Part model, mm, in its own coordinate system. A direction names the side the tool comes from. Coordinates: 2 decimals unless noted, no trailing zeros. Loops run counter-clockwise (first coordinate to the right, second up) from the corner with the lowest first, then second, coordinate; pieces in that order, holes last. Notation, with made-up numbers: (43.25, 51.5) - (67.25, 51.5) arc R13 ccw to (67.25, 75.5) - close; hole circle Ø8 at (-12.5, 14). An arc over 180 degrees is marked (long way). Use a Markdown table: item, result. Add a question column.
1. Wall check: probe 1 along X at (y, z) = (7.75, -19); probe 2 along X at (y, z) = (1.75, -3). Give the ranges that are in metal, low to high. Write a range as [from, to].
2. Drop flat-ended pins along their axis: pin 1 (1 mm diameter, centred on y = 0.5, z = 6.5, fed in from -X); pin 2 (0.5 mm diameter, centred on x = -2.5, y = 8, fed in from +Z); pin 3 (1 mm diameter, centred on x = 7.5, y = 8.5, fed in from +Z). Give the stop position or say it passes through.
3. Band-saw the part on B-B, the plane y = 4. Give the cut face in (x, z).
4. Band-saw the part on C-C, the plane x = 11.5. Give the cut face in (y, z).
5. Band-saw the part on A-A, the plane z = -16. Give the cut face in (x, y), plus the area to 3 significant figures.
6. 3-axis set-ups, long thin cutter, end or side, ignore diameter. For faces 4 (the flat face through (48.64, 4.36, 48.07)), 5 (the flat face through (45.543, 0.896, 46.075)), 6 (the cylindrical face through (-48.38, 0.342, 47.819)), 7 (the flat face through (0, 4, -63.184)), 8 (the flat face through (-45.543, 7.904, 46.075)): which of +Z, -Z, +X, -X, +Y, -Y reach the whole face in a straight line?
7. Pull direction Z, two halves, no side cores. Call faces 1 (the flat face through (45.543, 7.904, -46.075)), 2 (the cylindrical face through (-47.819, 0.342, -48.38)), 3 (the flat face through (-48.07, 4.36, 48.64)): pulls with the +Z half, pulls with the -Z half, needs draft (parallel to the pull), parting line crosses it, or undercut.
Autodesk Inventor part; units mm, degrees
ref_plane "작업 평면3" through (0, 4.4, 0) normal (0, -1, 0) x (1, 0, 0)
ref_plane "YZ Plane" through (0, 0, 0) normal (1, 0, 0) x (0, 1, 0)
ref_plane "XZ Plane" through (0, 0, 0) normal (0, 1, 0) x (-1, 0, 0)
sketch "스케치1" plane through (0, 0, 0) normal (0, 1, 0) x (-1, 0, 0)
  line L0 (-65.1838, 27) -> (-27, 65.1838)
  line L1 (-27, 65.1838) -> (27, 65.1838)
  line L2 (27, 65.1838) -> (65.1838, 27)
  line L3 (65.1838, 27) -> (65.1838, -27)
  line L4 (65.1838, -27) -> (27, -65.1838)
  line L5 (27, -65.1838) -> (-27, -65.1838)
  line L6 (-27, -65.1838) -> (-65.1838, -27)
  line L7 (-65.1838, -27) -> (-65.1838, 27)
  line L8 (68.3838, 28.3255) -> (68.3838, -28.3255)
  line L9 (68.3838, -28.3255) -> (28.3255, -68.3838)
  line L10 (28.3255, -68.3838) -> (-28.3255, -68.3838)
  line L11 (-28.3255, -68.3838) -> (-68.3838, -28.3255)
  line L12 (-68.3838, -28.3255) -> (-68.3838, 28.3255)
  line L13 (-68.3838, 28.3255) -> (-28.3255, 68.3838)
  line L14 (-28.3255, 68.3838) -> (28.3255, 68.3838)
  line L15 (28.3255, 68.3838) -> (68.3838, 28.3255)
  point P0 (0, 0)
  point P1 (0, 0)
  point P2 (0, 0)
  dimension "d0" = 54
  dimension "d1" = 3.2
extrude "돌출1" add sketch "스케치1" along normal blind 8.8 contours L0 L1 L2 L3 L4 L5 L6 L7 | L8 L9 L10 L11 L12 L13 L14 L15
sketch "스케치3" plane through (0, 0, 0) normal (0, -1, 0) x (1, 0, 0)
  line L0 (-26.8343, 64.7838) -> (26.8343, 64.7838)
  line L1 (26.8343, 64.7838) -> (64.7838, 26.8343)
  line L2 (64.7838, 26.8343) -> (64.7838, -26.8343)
  line L3 (64.7838, -26.8343) -> (26.8343, -64.7838)
  line L4 (26.8343, -64.7838) -> (-26.8343, -64.7838)
  line L5 (-26.8343, -64.7838) -> (-64.7838, -26.8343)
  line L6 (-64.7838, -26.8343) -> (-64.7838, 26.8343)
  line L7 (-64.7838, 26.8343) -> (-26.8343, 64.7838)
  line L8 (-27.6627, 66.7838) -> (27.6627, 66.7838)
  line L9 (27.6627, 66.7838) -> (66.7838, 27.6627)
  line L10 (66.7838, 27.6627) -> (66.7838, -27.6627)
  line L11 (66.7838, -27.6627) -> (27.6627, -66.7838)
  line L12 (27.6627, -66.7838) -> (-27.6627, -66.7838)
  line L13 (-27.6627, -66.7838) -> (-66.7838, -27.6627)
  line L14 (-66.7838, -27.6627) -> (-66.7838, 27.6627)
  line L15 (-66.7838, 27.6627) -> (-27.6627, 66.7838)
  line L16 (-28.3255, 68.3838) -> (28.3255, 68.3838)
  point P0 (0, 0)
  point P1 (0, 0)
  point P2 (0, 0)
  point P3 (0, 0)
  dimension "d9" = 2
  dimension "d144" = 1.6
extrude "돌출3" cut sketch "스케치3" against normal blind 1.2
sketch "스케치14" plane through (0, 0, 0) normal (0, -1, 0) x (1, 0, 0)
  line L0 (64.7838, 26.8343) -> (26.8343, 64.7838)
  line L1 (26.8343, 64.7838) -> (-26.8343, 64.7838)
  line L2 (-26.8343, 64.7838) -> (-64.7838, 26.8343)
  line L3 (-64.7838, 26.8343) -> (-64.7838, -26.8343)
  line L4 (-64.7838, -26.8343) -> (-26.8343, -64.7838)
  line L5 (-26.8343, -64.7838) -> (26.8343, -64.7838)
  line L6 (26.8343, -64.7838) -> (64.7838, -26.8343)
  line L7 (64.7838, -26.8343) -> (64.7838, 26.8343)
  point P0 (0, 0)
extrude "돌출16" cut sketch "스케치14" against normal blind 0.6
sketch "스케치15" plane through (0, 0.6, 0) normal (0, -1, 0) x (1, 0, 0)
  line L0 (-26.1716, 63.1838) -> (26.1716, 63.1838)
  line L1 (26.1716, 63.1838) -> (63.1838, 26.1716)
  line L2 (63.1838, 26.1716) -> (63.1838, -26.1716)
  line L3 (63.1838, -26.1716) -> (26.1716, -63.1838)
  line L4 (26.1716, -63.1838) -> (-26.1716, -63.1838)
  line L5 (-26.1716, -63.1838) -> (-63.1838, -26.1716)
  line L6 (-63.1838, -26.1716) -> (-63.1838, 26.1716)
  line L7 (-63.1838, 26.1716) -> (-26.1716, 63.1838)
  line L8 (-26.8343, 64.7838) -> (26.8343, 64.7838)
  point P0 (0, 0)
  point P1 (0, 0)
  dimension "d140" = 1.6
extrude "돌출17" cut sketch "스케치15" against normal up to surface (8.2 mm away)
ref_plane "작업 평면3" through (0, 4.4, 0) normal (0, -1, 0) x (1, 0, 0)
mirror "미러6" about plane through (0, 4.4, 0) normal (0, -1, 0) of "돌출3", "돌출16"
fillet "모깎기2" radius 1.2 16 edges at (0, 0, 68.3838) (-48.3546, 0, 48.3546) (-68.3838, 0, 0) (-48.3546, 0, -48.3546) (0, 0, -68.3838) (48.3546, 0, -48.3546) (68.3838, 0, 0) (48.3546, 0, 48.3546) (-48.3546, 8.8, 48.3546) (-68.3838, 8.8, 0) (-48.3546, 8.8, -48.3546) (0, 8.8, -68.3838) (48.3546, 8.8, -48.3546) (68.3838, 8.8, 0) (48.3546, 8.8, 48.3546) (0, 8.8, 68.3838)
properties part number "OV-PAM_ring_2"
Geometry check:
| question | item | result |
|---|---|---|
| 1 | probe 1 | x = [-68.37, -66.78], [-64.78, -63.18], [63.18, 64.78], [66.78, 68.37] |
| 1 | probe 2 | x = [-68.38, -63.18], [63.18, 68.38] |
| 2 | pin 1 | stops at x = -68.37 |
| 2 | pin 2 | stops at z = 68.37 |
| 2 | pin 3 | stops at z = 68.32 |
| 3 | outline | (-68.38, -28.33) - (-28.33, -68.38) - (28.33, -68.38) - (68.38, -28.33) - (68.38, 28.33) - (28.33, 68.38) - (-28.33, 68.38) - (-68.38, 28.33) - close; hole (-63.18, -26.17) - (-26.17, -63.18) - (26.17, -63.18) - (63.18, -26.17) - (63.18, 26.17) - (26.17, 63.18) - (-26.17, 63.18) - (-63.18, 26.17) - close |
| 4 | outline | (0, -67.18) arc R1.2 ccw to (1.2, -68.38) - (7.6, -68.38) arc R1.2 ccw to (8.8, -67.18) - (8.8, -66.78) - (7.6, -66.78) - (7.6, -64.78) - (8.2, -64.78) - (8.2, -63.18) - (0.6, -63.18) - (0.6, -64.78) - (1.2, -64.78) - (1.2, -66.78) - (0, -66.78) - close; (0, 66.78) - (1.2, 66.78) - (1.2, 64.78) - (0.6, 64.78) - (0.6, 63.18) - (8.2, 63.18) - (8.2, 64.78) - (7.6, 64.78) - (7.6, 66.78) - (8.8, 66.78) - (8.8, 67.18) arc R1.2 ccw to (7.6, 68.38) - (1.2, 68.38) arc R1.2 ccw to (0, 67.18) - close |
| 5 | outline | (-68.38, 1.2) arc R1.2 ccw to (-67.18, 0) - (-66.78, 0) - (-66.78, 1.2) - (-64.78, 1.2) - (-64.78, 0.6) - (-63.18, 0.6) - (-63.18, 8.2) - (-64.78, 8.2) - (-64.78, 7.6) - (-66.78, 7.6) - (-66.78, 8.8) - (-67.18, 8.8) arc R1.2 ccw to (-68.38, 7.6) - close; (63.18, 0.6) - (64.78, 0.6) - (64.78, 1.2) - (66.78, 1.2) - (66.78, 0) - (67.18, 0) arc R1.2 ccw to (68.38, 1.2) - (68.38, 7.6) arc R1.2 ccw to (67.18, 8.8) - (66.78, 8.8) - (66.78, 7.6) - (64.78, 7.6) - (64.78, 8.2) - (63.18, 8.2) - close |
| 5 | area | 76.8 mm^2 |
| 6 | face 4 | +Z, +X, +Y, -Y |
| 6 | face 5 | -Y |
| 6 | face 6 | +Z, -X, -Y |
| 6 | face 7 | +Y, -Y |
| 6 | face 8 | +Y |
| 7 | face 1 | undercut |
| 7 | face 2 | pulls with the -Z half |
| 7 | face 3 | pulls with the +Z half |
